The drawing under review shows one solid part. Ordinate dimensions are in mm from its lowest x, y, z. A direction names the side the tool comes from. Coordinates: 2 decimals unless noted, no trailing zeros. Write each loop counter-clockwise with the first axis right and the second up, starting at its lowest first coordinate (ties: lowest second). Pieces come first, ordered by that corner, then holes. Notation, with made-up numbers: (68, 22) -> (106, 22) arc R24 cw to (106, 48) -> close; hole circle Ø8 at (40.25, -4.75). An arc over 180 degrees is marked (long way). One line per question, with ' | ' between items. Start each with the question number.
Q1. Add section A-A on x = 10.16. State the section outline as (y, z) points, and give its area (3 significant figures).
Q2. For the marked faces 1, 2 and 3, list the 3-axis set-ups (+Z, -Z, +X, -X, +Y, -Y) from which the entire face can be reached by the end or side of a thin tool; tool diameter is ignored.
Q3. For P1, Ø1.5, axis at y = 3, z = 5, coming from the -X side; P2, Ø0.5, axis at y = 2, z = 9.5, coming from the +X side; P3, Ø1.5, axis at x = 3, z = 4, coming from the +Y side, all flat-tipped, find the tip position at first contact; note any pin that passes through.
Q4. Wall thickness on probe 1 along Z at (x, y) = (8, 2.2); probe 2 along Z at (x, y) = (10.16, 0.65); probe 3 along Y at (x, z) = (10.5, 4): over which ranges is each line inside the solid? List them lowest first.
Q5. Add section D-D on x = 4. State the section outline as (y, z) points, and give its area (3 significant figures).
Q6. Add section C-C on y = 0.9. State the section outline as (x, z) points, and give its area (3 significant figures).
Q7. Add section B-B on z = 12. State the section outline as (x, y) points.
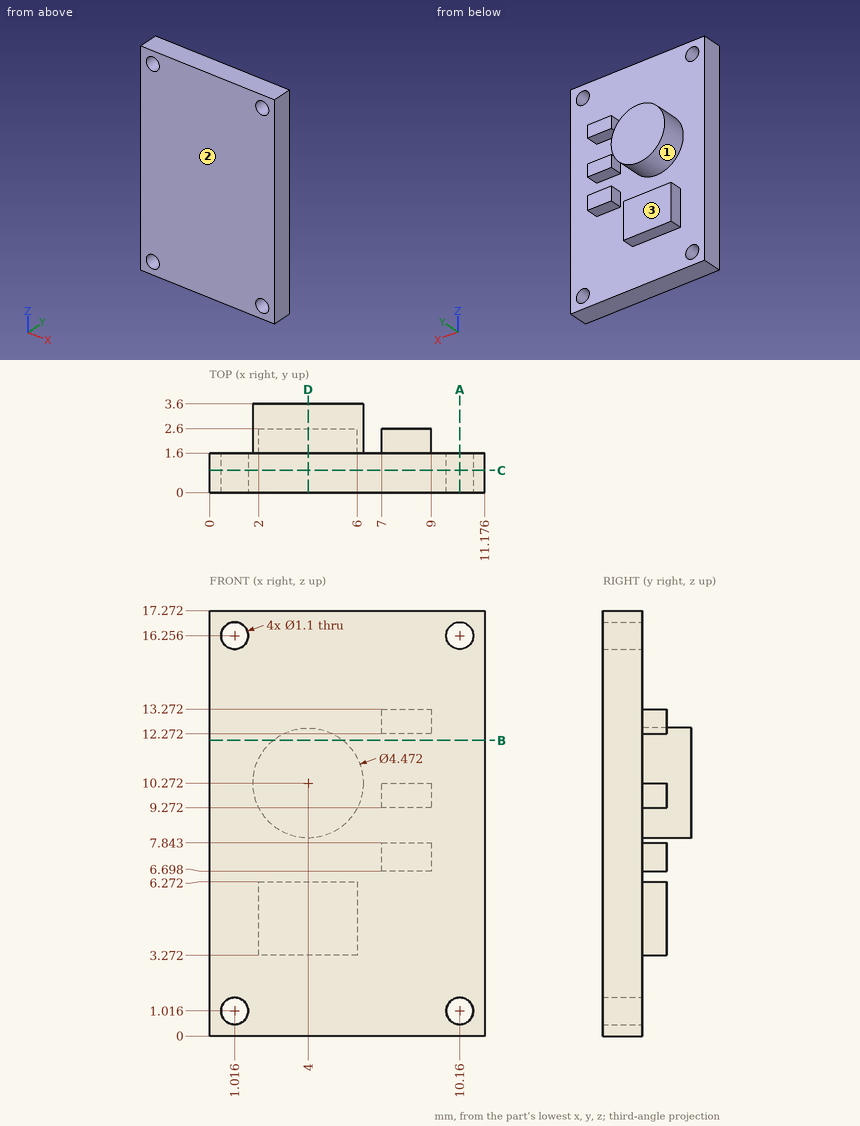
Output values:
1) outline: (0, 0) -> (1.6, 0) -> (1.6, 0.47) -> (0, 0.47) -> close; (0, 1.57) -> (1.6, 1.57) -> (1.6, 15.71) -> (0, 15.71) -> close; (0, 16.81) -> (1.6, 16.81) -> (1.6, 17.27) -> (0, 17.27) -> close | area: 24.1 mm2
2) face 1: +Y | face 2: +Z, -Z, +X, -X, -Y | face 3: -Z, +X, -X, +Y
3) P1: stops at x = 2 | P2: stops at x = 9 | P3: stops at y = 2.6
4) probe 1: z = 6.7 to 7.84, 9.27 to 10.27, 12.27 to 13.27 | probe 2: z = 0 to 0.47, 1.57 to 15.71, 16.81 to 17.27 | probe 3: y = 0 to 1.6
5) outline: (0, 0) -> (1.6, 0) -> (1.6, 3.27) -> (2.6, 3.27) -> (2.6, 6.27) -> (1.6, 6.27) -> (1.6, 8.04) -> (3.6, 8.04) -> (3.6, 12.51) -> (1.6, 12.51) -> (1.6, 17.27) -> (0, 17.27) -> close | area: 39.6 mm2
6) outline: (0, 0) -> (11.18, 0) -> (11.18, 17.27) -> (0, 17.27) -> close; hole circle Ø1.1 at (1.02, 1.02); hole circle Ø1.1 at (1.02, 16.26); hole circle Ø1.1 at (10.16, 1.02); hole circle Ø1.1 at (10.16, 16.26) | area: 189 mm2
7) outline: (0, 0) -> (11.18, 0) -> (11.18, 1.6) -> (5.42, 1.6) -> (5.42, 3.6) -> (2.58, 3.6) -> (2.58, 1.6) -> (0, 1.6) -> close
